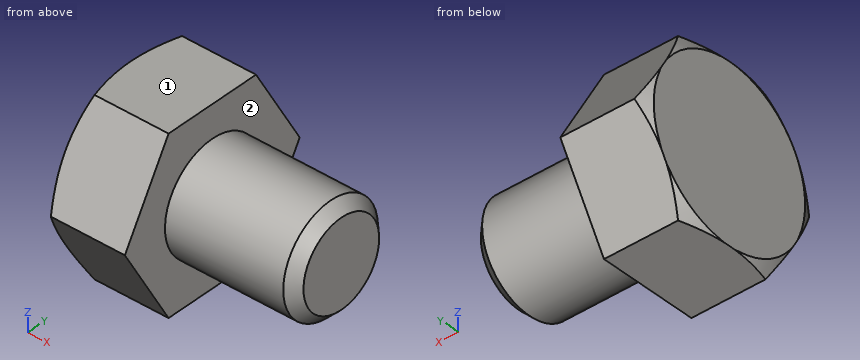
from build123d import *

# Parameters (mm, degrees)
SKETCH2_R       = 4.665127021
HEX_DIE_DEPTH   = 3.8
CHANFREIN1_SIZE = 0.5


with BuildPart() as part:
    # BodySke → Base-Revolve (revolve)
    with BuildSketch(Plane.XY, mode=Mode.PRIVATE) as base_revolve_sk:
        Polygon((3.8, 2.5), (3.8, 4.618937644), (0.357343816, 4.618937644), (0, 4), (0, 0), (9.8, 0), (9.8, 2.5), align=None)
    revolve(base_revolve_sk.sketch.rotate(Axis((-25.4, 0, 0), (1, 0, 0)), 90), axis=Axis((-25.4, 0, 0), (1, 0, 0)))

    # Sketch2 → Hex-Die (cut)
    with BuildSketch(Plane(origin=(0, 0, 0), x_dir=(0, 0, -1), z_dir=(1, 0, 0))):
        Circle(SKETCH2_R)
        Polygon((-4, 2.309401087), (0, 4.618802174), (4, 2.309401087), (4, -2.309401087), (0, -4.618802174), (-4, -2.309401087), align=None, mode=Mode.SUBTRACT)
    extrude(amount=HEX_DIE_DEPTH, mode=Mode.SUBTRACT)

    # Chanfrein1
    chanfrein1_edges = [part.edges().sort_by_distance(p)[0] for p in [
        (9.8, 0, -2.5),
    ]]
    chamfer(chanfrein1_edges, length=CHANFREIN1_SIZE)


solid = part.part
Geometry: final body of the model. Coordinates: model frame, mm. Face numbers are marked on the shaded views. A direction names the side the tool comes from. Give positions to 0.01 mm unless a question says otherwise; leave off trailing zeros. Write each loop counter-clockwise with the first axis right and the second up, starting at its lowest first coordinate (ties: lowest second). Pieces come first, ordered by that corner, then holes. Notation, with made-up numbers: (63.5, 55.5) - (115.5, 55.5) arc R15 ccw to (115.5, 64.5) - close; hole circle Ø10 at (-38, -31). An arc over 180 degrees is marked (long way). Return JSON: item names as keys, results as strings. Group by question number.
1) Set-up query: the marked faces 1 and 2. Return all of +Z, -Z, +X, -X, +Y, -Y with unobstructed straight access to the full face (end or side cutting, diameter ignored); none if empty.
2) First-contact query: P1, Ø4, axis at y = 3.5, z = 3, coming from the +X side; P2, Ø3, axis at x = 6, y = 0, coming from the -Z side. Flat tips, straight axial feed; report the tip coordinate or a pass-through.
3) Line query: line 1 (X direction, y = -3, z = 1); line 2 (Y direction, x = 5.25, z = 0); line 3 (Y direction, x = 5.75, z = 0.5). Output: solid intervals per line, ascending.
4) Section A-A on x = 8.25. Return the cut outline in (y, z).
5) Section B-B on x = 3. Return the cut outline in (y, z).
Filled in:
{
 "1": {"face 1": "+Z, +X, -X, +Y, -Y", "face 2": "+X"},
 "2": {"P1": "stops at x = 3.8", "P2": "stops at z = -2.5"},
 "3": {"line 1": "x = 0 to 3.8", "line 2": "y = -2.5 to 2.5", "line 3": "y = -2.45 to 2.45"},
 "4": {"outline": "circle Ø5 at (0, 0)"},
 "5": {"outline": "(-4.62, 0) - (-2.31, -4) - (2.31, -4) - (4.62, 0) - (2.31, 4) - (-2.31, 4) - close"}
}
